Here's how the part is built. I have some questions about the finished solid (model axes, mm). Face numbers are marked on the shaded views. A direction names the side the tool comes from. Round coordinates to 2 decimals unless told otherwise and drop trailing zeros. Loops run counter-clockwise (first coordinate to the right, second up) from the corner with the lowest first, then second, coordinate; pieces in that order, holes last. Notation, with made-up numbers: M 53,52 L 93,52 A32 ccw 93,86 Z; hole C -13.75,-36.5 d7. An arc over 180 degrees is marked long. Put each result on its own line as item: value. Start each with the question number.
```python
from build123d import *

# Parameters (mm, degrees)
F0_R     = 25
F0_R_2   = 5
F0_R_3   = 75
F1_DEPTH = 20
F2_DEPTH = 60


with BuildPart() as f1:
    # F0 (on Front) → F1 (new body)
    with BuildSketch(Plane.XZ):
        with BuildLine():
            ThreePointArc((86.129578, 185.121394), (0, 238.845987), (-86.129578, 185.121394))
            Line((-86.129578, 185.121394), (-138.221827, 64.268738))
            ThreePointArc((-138.221827, 64.268738), (0, -152.432753), (138.221827, 64.268738))
            Line((138.221827, 64.268738), (86.129578, 185.121394))
        make_face()
        Circle(F0_R, mode=Mode.SUBTRACT)
        with Locations((-63.50091, 87.336254)):
            Circle(F0_R_2, mode=Mode.SUBTRACT)
        with Locations((-83.826575, 152.82513)):
            Circle(F0_R_2, mode=Mode.SUBTRACT)
        with Locations((-56.082384, 206.025317)):
            Circle(F0_R_2, mode=Mode.SUBTRACT)
        with Locations((63.50091, 87.336254)):
            Circle(F0_R_2, mode=Mode.SUBTRACT)
        with Locations((0, 142.943576)):
            Circle(F0_R_3, mode=Mode.SUBTRACT)
        with Locations((0, 227.350565)):
            Circle(F0_R_2, mode=Mode.SUBTRACT)
        with Locations((56.082384, 206.025317)):
            Circle(F0_R_2, mode=Mode.SUBTRACT)
        with Locations((83.826575, 152.82513)):
            Circle(F0_R_2, mode=Mode.SUBTRACT)
    extrude(amount=F1_DEPTH)

    # F0 (on Front) → F2 (join)
    with BuildSketch(Plane.XZ):
        with BuildLine():
            Line((145.524237, 67.537877), (93.401044, 188.462319))
            ThreePointArc((93.401044, 188.462319), (0, 246.845987), (-93.401044, 188.462319))
            Line((-93.401044, 188.462319), (-145.524237, 67.537877))
            ThreePointArc((-145.524237, 67.537877), (0, -160.432753), (145.524237, 67.537877))
        make_face()
        with BuildLine():
            Line((-138.221827, 64.268738), (-86.129578, 185.121394))
            ThreePointArc((-86.129578, 185.121394), (0, 238.845987), (86.129578, 185.121394))
            Line((86.129578, 185.121394), (138.221827, 64.268738))
            ThreePointArc((138.221827, 64.268738), (0, -152.432753), (-138.221827, 64.268738))
        make_face(mode=Mode.SUBTRACT)
    extrude(amount=F2_DEPTH)


solid = f1.part
```
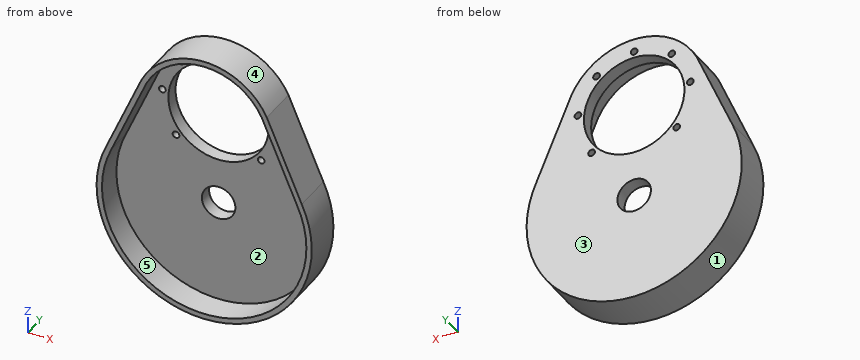
1) Suppose I cut it at D-D (z = -88.5). Write out the boundary of the cut face in (x, y), plus the area to 3 significant figures.
2) If we mould it in two halves opening along Z, with no side actions, what happens to the marked faces 1, 2 and 3? For each: pulls with the +Z half, pulls with the -Z half, needs draft (parallel to the pull), parting line crosses it, or undercut.
3) I'm going to push flat-ended pins straight in: P1, Ø2, axis at x = -49.5, y = -13, coming from the -Z side; P2, Ø8, axis at x = 76, y = -16.5, coming from the +Z side; P3, Ø1.5, axis at y = -33, z = 113, coming from the -X side; P4, Ø8, axis at x = -56.08, z = 206.03, coming from the +Y side. Where does each tip first touch, or does it pass through?
4) Suppose I cut it at C-C (x = -37). Write out the boundary of the cut face in (y, z), plus the area to 3 significant figures.
5) On a 3-axis mill with a long thin cutter (end or side, diameter ignored), from which of +Z, -Z, +X, -X, +Y, -Y can I reach the whole of each face in a straight line? I mean the marked faces 4 and 5. Say none if no direction works.
6) If I drill on probe 1 along X at (y, z) = (-5.5, 155.5); probe 2 along Y at (x, z) = (73, 1.5); probe 3 along Z at (x, y) = (57.5, -41), over which ranges is the centre line in solid material (lowest first)? Write a range as from..to.
7) Suppose I cut it at A-A (x = 0). Write out the boundary of the cut face in (y, z), plus the area to 3 significant figures.
8) Suppose I cut it at B-B (z = 0). Write out the boundary of the cut face in (x, y).
Results are:
1. outline: M -133.81,-60 L -124.11,-60 L -124.11,-20 L 124.11,-20 L 124.11,-60 L 133.81,-60 L 133.81,0 L -133.81,0 Z
1. area: 6,130 mm²
2. face 1: parting line crosses it
2. face 2: undercut
2. face 3: needs draft
3. P1: z = -152.93
3. P2: z = 217.85
3. P3: x = -126.25
3. P4: through
4. outline: M -60,-156.11 L 0,-156.11 L 0,77.71 L -20,77.71 L -20,-147.87 L -60,-147.87 Z; M -60,231.42 L -20,231.42 L -20,208.18 L 0,208.18 L 0,240.03 L -60,240.03 Z
4. area: 5,990 mm²
5. face 4: +Z, +Y, -Y
5. face 5: -Y
6. probe 1: -107.61..-88.05, -79.6..-73.94, 73.94..79.6, 88.05..107.61
6. probe 2: -20..0
6. probe 3: -149.77..-141.17, 219.7..229.49
7. outline: M -60,-160.43 L 0,-160.43 L 0,-25 L -20,-25 L -20,-152.43 L -60,-152.43 Z; M -60,238.85 L -20,238.85 L -20,232.35 L 0,232.35 L 0,246.85 L -60,246.85 Z; M -20,25 L 0,25 L 0,67.94 L -20,67.94 Z; M -20,217.94 L 0,217.94 L 0,222.35 L -20,222.35 Z
7. area: 4,590 mm²
8. outline: M -160.43,-60 L -152.43,-60 L -152.43,-20 L -25,-20 L -25,0 L -160.43,0 Z; M 25,-20 L 152.43,-20 L 152.43,-60 L 160.43,-60 L 160.43,0 L 25,0 Z
